For this review, take the finished solid that the model builds, in its own axes (mm). Round coordinates to 2 decimals unless told otherwise and drop trailing zeros. Write each loop counter-clockwise with the first axis right and the second up, starting at its lowest first coordinate (ties: lowest second). Pieces come first, ordered by that corner, then holes. Notation, with made-up numbers: M 56.25,-30.75 L 90.25,-30.75 A34 cw 90.25,0.25 Z; hole C -2,8.25 d3. An arc over 180 degrees is marked long. Write each question's results on one line, items separated by ' | '. Start each with the question number.
```python
from build123d import *

# Parameters (mm, degrees)
CROQUIS1_W              = 53
CROQUIS1_H              = 45
SALIENTE_EXTRUIR1_DEPTH = 10
CROQUIS2_R              = 0.8
CORTAR_EXTRUIR1_DEPTH   = 10
CROQUIS3_R              = 1.45
CORTAR_EXTRUIR2_DEPTH   = 10
CROQUIS4_R              = 3
CORTAR_EXTRUIR3_DEPTH   = 5
CROQUIS5_R              = 1.45
CORTAR_EXTRUIR4_DEPTH   = 10


with BuildPart() as part:
    # Croquis1 → Saliente-Extruir1 (new body)
    with BuildSketch(Plane.XY):
        with Locations((8.456656727, -2.798833819)):
            Rectangle(CROQUIS1_W, CROQUIS1_H)
    extrude(amount=SALIENTE_EXTRUIR1_DEPTH)

    # Croquis2 → Cortar-Extruir1 (cut)
    with BuildSketch(Plane.XY.offset(10)):
        with Locations((6.286656727, -19.898833819)):
            Circle(CROQUIS2_R)
        with Locations((10.626656727, -19.898833819)):
            Circle(CROQUIS2_R)
    extrude(amount=-CORTAR_EXTRUIR1_DEPTH, mode=Mode.SUBTRACT)

    # Croquis3 → Cortar-Extruir2 (cut)
    with BuildSketch(Plane.XY.offset(10)):
        with Locations((13.356656727, 6.701166181)):
            Circle(CROQUIS3_R)
        with Locations((3.556656727, 6.701166181)):
            Circle(CROQUIS3_R)
    extrude(amount=-CORTAR_EXTRUIR2_DEPTH, mode=Mode.SUBTRACT)

    # Croquis4 → Cortar-Extruir3 (cut)
    with BuildSketch(Plane.XY.offset(10)):
        with Locations((3.556656727, 6.701166181)):
            Circle(CROQUIS4_R)
        with Locations((13.356656727, 6.701166181)):
            Circle(CROQUIS4_R)
    extrude(amount=-CORTAR_EXTRUIR3_DEPTH, mode=Mode.SUBTRACT)

    # Croquis5 → Cortar-Extruir4 (cut)
    with BuildSketch(Plane.XY.offset(10)):
        with Locations((-13.043343273, -2.798833819)):
            Circle(CROQUIS5_R)
        with Locations(Location((29.956656727, -2.798833819, 0), (0, 0, 180))):
            Circle(CROQUIS5_R)
    extrude(amount=-CORTAR_EXTRUIR4_DEPTH, mode=Mode.SUBTRACT)


solid = part.part
```
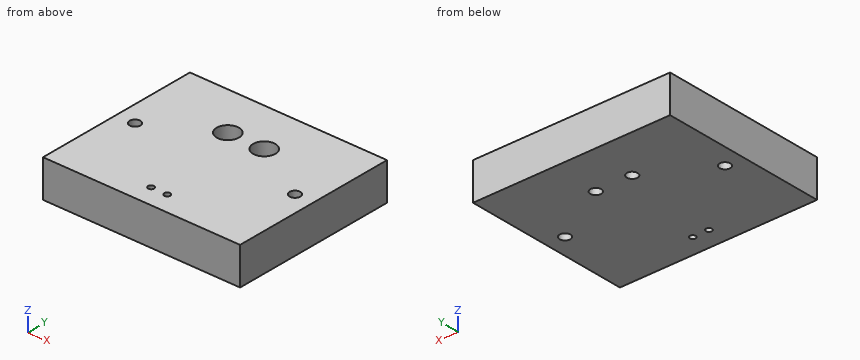
Item 1: For probe 1 along X at (y, z) = (-3, 5); probe 2 along Y at (x, z) = (-13, 8); probe 3 along X at (y, z) = (6.5, 8.25), list the stretches that pass through material, from the lowest coordinate up.
Item 2: Insertion check: P1, Ø1.4, axis at x = 6.29, y = -19.9, coming from the -Z side; P2, Ø5, axis at x = 3.5, y = 6.5, coming from the +Z side. Each pin has a flat end and moves straight along its axis. Give the tip position at first contact, or say it passes through.
Item 3: We need section A-A on x = 30. State the section outline as (y, z) points.
Item 4: We need section C-C on x = 14. State the section outline as (y, z) points.
Item 5: We need section B-B on z = 6.5. State the section outline as (x, y) points, then the cut area to 3 significant figures.
Numbers:
1) probe 1: x = -18.04 to -14.48, -11.61 to 28.52, 31.39 to 34.96 | probe 2: y = -25.3 to -4.25, -1.35 to 19.7 | probe 3: x = -18.04 to 0.56, 6.55 to 10.36, 16.35 to 34.96
2) P1: passes through | P2: stops at z = 5
3) outline: M -25.3,0 L -4.25,0 L -4.25,10 L -25.3,10 Z; M -1.35,0 L 19.7,0 L 19.7,10 L -1.35,10 Z
4) outline: M -25.3,0 L 5.4,0 L 5.4,5 L 3.77,5 L 3.77,10 L -25.3,10 Z; M 8,0 L 19.7,0 L 19.7,10 L 9.63,10 L 9.63,5 L 8,5 Z
5) outline: M -18.04,-25.3 L 34.96,-25.3 L 34.96,19.7 L -18.04,19.7 Z; hole C -13.04,-2.8 d2.9; hole C 3.56,6.7 d6; hole C 6.29,-19.9 d1.6; hole C 10.63,-19.9 d1.6; hole C 13.36,6.7 d6; hole C 29.96,-2.8 d2.9 | area: 2,310 mm^2
